Model file for the job. Use its own axes, mm. A direction names the side the tool comes from. Give positions to 0.01 mm unless a question says otherwise; leave off trailing zeros. Write each loop counter-clockwise with the first axis right and the second up, starting at its lowest first coordinate (ties: lowest second). Pieces come first, ordered by that corner, then holes. Notation, with made-up numbers: (17, -34.75) - (42, -34.75) arc R19 ccw to (42, -26.75) - close; hole circle Ø7 at (-39, 20). An arc over 180 degrees is marked (long way). One line per item, written item: value. Start each with the question number.
(1) Drop flat-ended pins along their axis: P1, Ø0.5, axis at x = 3, z = -3, coming from the +Y side; P2, Ø5, axis at x = 3.5, y = 42, coming from the -Z side; P3, Ø0.5, axis at y = 15, z = -3, coming from the -X side; P4, Ø1, axis at y = 39, z = -1, coming from the -X side. Give the stop position or say it passes through.
(2) Probe L1, parallel to Y at x = 5, z = 0.7; L2, parallel to Y at x = 3, z = -4; L3, parallel to Z at x = 5.5, y = 34. List the from-to ranges inside material, lowest first.
(3) Mould opens along X. For faces 5 (the face through (6.5, 15, -2)), 6 (the face through (4.5, 15, -2)), 7 (the face through (3, 15.5, -2)), 8 (the face through (2.5, 15, -2)) say: pulls with the +X half, pulls with the -X half, needs draft (parallel to the pull), parting line crosses it, or undercut.
(4) Cut at A-A, the plane z = -2.75. List the corners of the cut face in (x, y), and give its area (3 significant figures).
(5) 3-axis set-ups, long thin cutter, end or side, ignore diameter. For faces 1 (the face through (7.5, 15, -2)), 2 (the face through (5.5, 15, -2)), 3 (the face through (3, 14.5, -2)), 4 (the face through (5, 40, -1)): which of +Z, -Z, +X, -X, +Y, -Y reach the whole face in a straight line?
(6) Cut at C-C, the plane x = 5. List the corners of the cut face in (y, z), and give its area (4 significant figures).
(7) Cut at D-D, the plane z = 2. List the corners of the cut face in (x, y), and give its area (3 significant figures).
(8) Cut at B-B, the plane y = 3. List the corners of the cut face in (x, z).
from build123d import *

# Parameters (mm, degrees)
SKETCH_2_W      = 10
SKETCH_2_H      = 40
SKETCH_2_R      = 1.5
EXTRUDE_1_DEPTH = 1.5
SKETCH_3_3_W    = 6
SKETCH_3_3_H    = 6
EXTRUDE_3_DEPTH = 6
SKETCH_3_4_W    = 6
SKETCH_3_4_H    = 2
EXTRUDE_4_DEPTH = 2
SKETCH_4_W      = 1
SKETCH_4_H      = 1
EXTRUDE_5_DEPTH = 4
SKETCH_6_W      = 6
SKETCH_6_H      = 4
EXTRUDE_6_DEPTH = 7.5


with BuildPart() as part:
    # 草圖2 → 填料-伸長1 (new body)
    with BuildSketch(Plane.XY):
        with Locations((5, 20)):
            Rectangle(SKETCH_2_W, SKETCH_2_H)
        with Locations((5, 3)):
            Circle(SKETCH_2_R, mode=Mode.SUBTRACT)
    extrude(amount=EXTRUDE_1_DEPTH)

    # 草圖3<3> → 填料-伸長3 (add)
    with BuildSketch(Plane.XY.offset(1.5)):
        with Locations((5, 20)):
            Rectangle(SKETCH_3_3_W, SKETCH_3_3_H)
    extrude(amount=-EXTRUDE_3_DEPTH)

    # 草圖3<4> → 填料-伸長4 (add)
    with BuildSketch(Plane.XY.offset(1.5)):
        with Locations((5, 15)):
            Rectangle(SKETCH_3_4_W, SKETCH_3_4_H)
    extrude(amount=-EXTRUDE_4_DEPTH)

    # 草圖4 → 填料-伸長5 (add)
    with BuildSketch(Plane(origin=(0, 0, -0.5), x_dir=(-1, 0, 0), z_dir=(0, 0, -1))):
        with Locations((-5, 15)):
            Rectangle(SKETCH_4_W, SKETCH_4_H)
        with Locations((-7, 15)):
            Rectangle(SKETCH_4_W, SKETCH_4_H)
        with Locations((-3, 15)):
            Rectangle(SKETCH_4_W, SKETCH_4_H)
    extrude(amount=EXTRUDE_5_DEPTH)

    # 草圖6 → 填料-伸長6 (add)
    with BuildSketch(Plane(origin=(0, 40, 0), x_dir=(1, 0, 0), z_dir=(0, 1, 0))):
        with Locations((5, -0.75)):
            Rectangle(SKETCH_6_W, SKETCH_6_H)
    extrude(amount=EXTRUDE_6_DEPTH)


solid = part.part
Answers follow:
1. P1: stops at y = 23
1. P2: stops at z = -1.25
1. P3: stops at x = 2.5
1. P4: passes through
2. L1: y = 0 to 1.5, 4.5 to 47.5
2. L2: y = 14.5 to 15.5, 17 to 23
2. L3: z = 0 to 1.5
3. face 5: undercut
3. face 6: undercut
3. face 7: needs draft
3. face 8: pulls with the -X half
4. outline: (2, 17) - (8, 17) - (8, 23) - (2, 23) - close; (2.5, 14.5) - (3.5, 14.5) - (3.5, 15.5) - (2.5, 15.5) - close; (4.5, 14.5) - (5.5, 14.5) - (5.5, 15.5) - (4.5, 15.5) - close; (6.5, 14.5) - (7.5, 14.5) - (7.5, 15.5) - (6.5, 15.5) - close
4. area: 39.0 mm²
5. face 1: -Z, +X, -Y
5. face 2: -Z, -Y
5. face 3: -Z, +X, -X, -Y
5. face 4: -Z, +X, -X
6. outline: (0, 0) - (1.5, 0) - (1.5, 1.5) - (0, 1.5) - close; (4.5, 0) - (14, 0) - (14, -0.5) - (14.5, -0.5) - (14.5, -4.5) - (15.5, -4.5) - (15.5, -0.5) - (16, -0.5) - (16, 0) - (17, 0) - (17, -4.5) - (23, -4.5) - (23, 0) - (40, 0) - (40, -1.25) - (47.5, -1.25) - (47.5, 2.75) - (40, 2.75) - (40, 1.5) - (4.5, 1.5) - close
6. area: 117.5 mm²
7. outline: (2, 40) - (8, 40) - (8, 47.5) - (2, 47.5) - close
7. area: 45.0 mm²
8. outline: (0, 0) - (3.5, 0) - (3.5, 1.5) - (0, 1.5) - close; (6.5, 0) - (10, 0) - (10, 1.5) - (6.5, 1.5) - close
